Read the model definition and answer for the solid it produces. Units are mm, in the model's axes. A direction names the side the tool comes from. Coordinates: 2 decimals unless noted, no trailing zeros. Write each loop counter-clockwise with the first axis right and the second up, starting at its lowest first coordinate (ties: lowest second). Pieces come first, ordered by that corner, then holes. Notation, with made-up numbers: (-29, 47) -> (-25, 47) arc R24 ccw to (-25, 69) -> close; hole circle Ø2 at (-4.5, -8.5). An arc over 180 degrees is marked (long way). One line per item, written item: value. Start each with the question number.
1. Consider line 1 along Y through (x, z) = (-4.5, 3.5); line 2 along X through (y, z) = (4.5, -0.5); line 3 along Z through (x, y) = (-1.25, 4). Determine where each line is inside the solid, lowest interval first.
2. Find section A-A, the plane y = 11.25. Write down the section's boundary in (x, z), and give its area (3 significant figures).
3. For a pull along Y with two mould halves and no side action, classify faces 4 (the cylindrical face through (-2.52, 10.26, -0.22)), 5 (the flat face through (1, 12, 0)), 6 (the cylindrical face through (2.48, 10.26, -0.22)), 7 (the flat face through (0, 8.5, 0)) as pulls with the +Y half, pulls with the -Y half, needs draft (parallel to the pull), parting line crosses it, or undercut.
4. Given P1, Ø1.7, axis at y = 11, z = -0.13, coming from the +X side; P2, Ø0.6, axis at x = 0.5, z = -1.5, coming from the +Y side; P3, Ø3, axis at x = 2, y = 3, coming from the +Z side, each flat-ended and moving along its own axis, determine where each tip first touches the part or whether it passes through.
5. For faces 1 (the conical face through (3.2, 13.8, 0.1)), 2 (the cylindrical face through (-1.532, 10.465, 3.695)), 3 (the flat face through (-1, 12, 0)), determine the directions among +Z, -Z, +X, -X, +Y, -Y from which every point of the face is accessible in a straight line to the end or side of a thin tool.
6. Find section D-D, the plane y = 7.5. Write down the section's boundary in (x, z).
7. Find section B-B, the plane x = 0. Write down the section's boundary in (y, z), and give its area (3 significant figures).
8. Find section C-C, the plane z = 0. Write down the section's boundary in (x, y), and give its area (3 significant figures).
```python
from build123d import *

# Parameters (mm, degrees)
SKETCH1_R               = 6.5
BOSS_EXTRUDE1_DEPTH     = 8
SKETCH2_R               = 4
BOSS_EXTRUDE2_DEPTH     = 6
SKETCH3_W               = 2
SKETCH3_H               = 9
CUT_EXTRUDE1_DEPTH      = 5.5
CHAMFER1_SIZE           = 1
CHAMFER2_SIZE           = 1
CUT_EXTRUDE3_DEPTH      = 5.5
CUT_EXTRUDE3_DEPTH_BACK = 5.5
SKETCH5_R               = 0.75


with BuildPart() as part:
    # Sketch1 → Boss-Extrude1 (new body)
    with BuildSketch(Plane(origin=(0, 0, 0), x_dir=(1, 0, 0), z_dir=(0, 1, 0))):
        with Locations(Location((0, 0, 0), (0, 0, 270))):
            Circle(SKETCH1_R)
    extrude(amount=BOSS_EXTRUDE1_DEPTH)

    # Sketch2 → Boss-Extrude2 (add)
    with BuildSketch(Plane(origin=(0, 8, 0), x_dir=(1, 0, 0), z_dir=(0, 1, 0))):
        with Locations(Location((0, 0, 0), (0, 0, 270))):
            Circle(SKETCH2_R)
    extrude(amount=BOSS_EXTRUDE2_DEPTH)

    # Sketch3 → Cut-Extrude1 (cut)
    with BuildSketch(Plane(origin=(0, 14, 0), x_dir=(1, 0, 0), z_dir=(0, 1, 0))):
        Rectangle(SKETCH3_W, SKETCH3_H)
    extrude(amount=-CUT_EXTRUDE1_DEPTH, mode=Mode.SUBTRACT)

    # Chamfer1
    chamfer1_edges = [part.edges().sort_by_distance(p)[0] for p in [
        (4, 14, 0),
    ]]
    chamfer(chamfer1_edges, length=CHAMFER1_SIZE)

    # Chamfer2
    chamfer2_edges = [part.edges().sort_by_distance(p)[0] for p in [
        (-4, 14, 0),
    ]]
    chamfer(chamfer2_edges, length=CHAMFER2_SIZE)

    # Sketch5 → Cut-Extrude3 (cut, two sides: drawn at the far end of the back side and taken through both)
    with BuildSketch(Plane(origin=(0, 0, 0), x_dir=(0, 0, -1), z_dir=(1, 0, 0)).offset(-CUT_EXTRUDE3_DEPTH_BACK)):
        with Locations(Location((0.127016654, 11.002690078, 0), (0, 0, 180))):
            Circle(SKETCH5_R)
    extrude(amount=CUT_EXTRUDE3_DEPTH + CUT_EXTRUDE3_DEPTH_BACK, mode=Mode.SUBTRACT)


solid = part.part
```
Answer block:
1. line 1: y = 0 to 8
1. line 2: x = -6.48 to 6.48
1. line 3: z = -6.38 to 6.38
2. outline: (-3.96, 0.58) -> (-1, 0.58) -> (-1, 3.87) arc R4 ccw to start; (-3.91, -0.84) arc R4 ccw to (-1, -3.87) -> (-1, -0.84) -> close; (1, -3.87) arc R4 ccw to (3.91, -0.84) -> (1, -0.84) -> close; (1, 0.58) -> (3.96, 0.58) arc R4 ccw to (1, 3.87) -> close
2. area: 26.0 mm2
3. face 4: undercut
3. face 5: needs draft
3. face 6: undercut
3. face 7: pulls with the +Y half
4. P1: stops at x = 4
4. P2: stops at y = 8.5
4. P3: stops at z = 6.48
5. face 1: +X, +Y
5. face 2: +Y
5. face 3: +Z, -Z, +Y
6. outline: circle Ø13 at (0, 0)
7. outline: (0, -6.5) -> (8, -6.5) -> (8, -4) -> (8.5, -4) -> (8.5, 4) -> (8, 4) -> (8, 6.5) -> (0, 6.5) -> close
7. area: 108 mm2
8. outline: (-6.5, 0) -> (6.5, 0) -> (6.5, 8) -> (4, 8) -> (4, 10.26) -> (1, 10.26) -> (1, 8.5) -> (-1, 8.5) -> (-1, 10.26) -> (-4, 10.26) -> (-4, 8) -> (-6.5, 8) -> close; (-4, 11.74) -> (-1, 11.74) -> (-1, 14) -> (-3, 14) -> (-4, 13) -> close; (1, 11.74) -> (4, 11.74) -> (4, 13) -> (3, 14) -> (1, 14) -> close
8. area: 131 mm2
